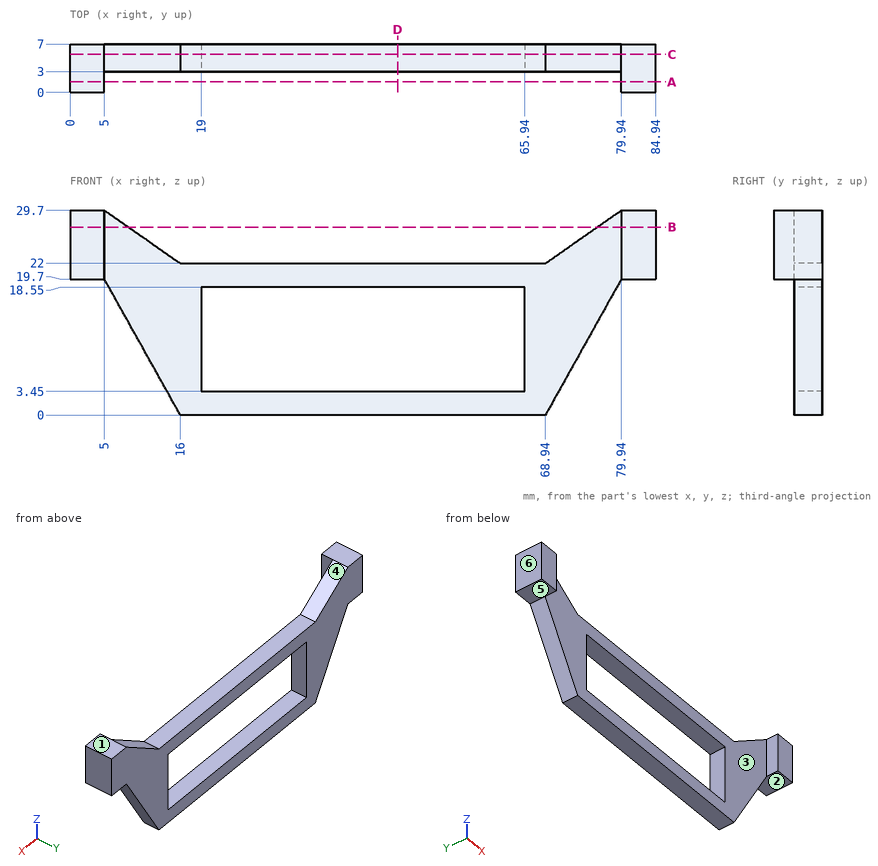
Verification items for this drawing (mm, ordinates from the low corner). A direction names the side the tool comes from. Give positions to 0.01 mm unless a question says otherwise; leave off trailing zeros. Loops run counter-clockwise (first coordinate to the right, second up) from the corner with the lowest first, then second, coordinate; pieces in that order, holes last.
(1) Section check B-B on z = 27.25. Record the cut outline in (x, y), then the cut area to 3 significant figures.
From the geometry:
outline: (0, 0) - (5, 0) - (5, 3) - (8.5, 3) - (8.5, 7) - (0, 7) - close; (76.44, 3) - (79.94, 3) - (79.94, 0) - (84.94, 0) - (84.94, 7) - (76.44, 7) - close
area: 98.0 mm2
(2) Section check C-C on y = 5.5. Record the cut outline in (x, z).
From the geometry:
outline: (0, 19.7) - (5, 19.7) - (16, 0) - (68.94, 0) - (79.94, 19.7) - (84.94, 19.7) - (84.94, 29.7) - (79.94, 29.7) - (68.94, 22) - (16, 22) - (5, 29.7) - (0, 29.7) - close; hole (19, 3.45) - (65.94, 3.45) - (65.94, 18.55) - (19, 18.55) - close
(3) Depth check by flat-ended pin: pin 1 Ø2 at (x, y) = (46.5, 5.5) entering from +Z; pin 2 Ø2 at (y, z) = (4.5, 8) entering from -X; pin 3 Ø2.5 at (x, y) = (3, 4) entering from -Z. Enter the tip coordinate at first touch or a pass-through.
From the geometry:
pin 1: stops at z = 22
pin 2: stops at x = 10.97
pin 3: stops at z = 19.7
(4) Thickness scan on L1, parallel to Z at x = 65, y = 5; L2, parallel to X at y = 2.75, z = 26; L3, parallel to Y at x = 34, z = 19. Record the ranges inside material, lowest first.
From the geometry:
L1: z = 0 to 3.45, 18.55 to 22
L2: x = 0 to 5, 79.94 to 84.94
L3: y = 3 to 7
(5) Section check D-D on x = 47.5. Record the cut outline in (y, z), then the cut area to 3 significant figures.
From the geometry:
outline: (3, 0) - (7, 0) - (7, 3.45) - (3, 3.45) - close; (3, 18.55) - (7, 18.55) - (7, 22) - (3, 22) - close
area: 27.6 mm2
(6) Section check A-A on y = 1.5. Record the cut outline in (x, z).
From the geometry:
outline: (0, 19.7) - (5, 19.7) - (5, 29.7) - (0, 29.7) - close; (79.94, 19.7) - (84.94, 19.7) - (84.94, 29.7) - (79.94, 29.7) - close
(7) Set-up check for the marked faces 1, 2 and 3: record each of +Z, -Z, +X, -X, +Y, -Y from which the full face is reachable in a straight line by a thin tool's end or side.
From the geometry:
face 1: +Z, +X, -X, +Y, -Y
face 2: -Z, +X, +Y, -Y
face 3: +Z, -Z, -Y
(8) Release check for a two-part mould opening along X. For the marked faces 4, 5 and 6 record: released by +X, released by -X, zero draft, split by the parting line, or undercut.
From the geometry:
face 4: undercut
face 5: zero draft
face 6: released by -X
